For this review, take the finished solid that the model builds, in its own axes (mm). Face numbers are marked on the shaded views. A direction names the side the tool comes from. Give positions to 0.01 mm unless a question says otherwise; leave off trailing zeros. Order: outer loops, then holes, each group sorted by start corner. A loop starts at its lowest first (then second) coordinate and runs counter-clockwise, first axis right, second up. Notation, with made-up numbers: (42.5, -3.5) -> (92.5, -3.5) arc R20 ccw to (92.5, 6.5) -> close; hole circle Ø8 at (74.5, 39). An arc over 180 degrees is marked (long way). Return JSON: item names as keys, results as strings. Group by question number.
1) For the marked faces 1, 2 and 3, list the 3-axis set-ups (+Z, -Z, +X, -X, +Y, -Y) from which the entire face can be reached by the end or side of a thin tool; tool diameter is ignored.
2) Add section A-A (y = 0). State how many separate pieces and enclosed holes the cut face has, then the cut area to 3 significant figures.
3) Add section B-B (x = 0). Give the boundary of the cut face in (y, z) (3 decimals).
4) To check wall thickness, follow line 1 along Y through (x, z) = (0, -9) (3 decimals); line 2 along Y through (x, z) = (10, 16); line 3 along X through (y, z) = (-8, -22). State the ranges of each line that lie inside material, in increasing order.
5) The part is to be moulded in two halves that separate along X. For the marked faces 4, 5, 6 and 7, say which applies: released by +X, released by -X, zero draft, split by the parting line, or undercut.
6) Insertion check: P1, Ø4, axis at x = -29.5, y = 18, coming from the +Z side; P2, Ø14.5, axis at x = 17.46, y = 30.25, coming from the -Z side; P3, Ø1, axis at y = 10, z = 14.5, coming from the -X side. Each pin has a flat end and moves straight along its axis. Give the tip position at first contact, or say it passes through.
from build123d import *

# Parameters (mm, degrees)
F_3_8_0_5_DIAMETER_HOLE1_D = 12.7
CIRPATTERN1_COUNT          = 6


with BuildPart() as part:
    # Sketch1 → Revolve1 (revolve)
    with BuildSketch(Plane(origin=(0, 0, 0), x_dir=(0, 0, -1), z_dir=(1, 0, 0)), mode=Mode.PRIVATE) as revolve1_sk:
        Polygon((-29.3497, 12.7), (29.3497, 12.7), (29.3497, 17.907), (4.826, 22.225), (4.826, 47.625), (22.225, 47.625), (22.225, 50.8), (-22.225, 50.8), (-22.225, 47.625), (-4.826, 47.625), (-4.826, 22.225), (-29.3497, 17.907), align=None)
    revolve(revolve1_sk.sketch.rotate(Axis((0, 0, 50.332885059), (0, 0, -1)), 90), axis=Axis((0, 0, 50.332885059), (0, 0, -1)))

    # 3/8 (0.5) Diameter Hole1 (through all)
    with Locations(Plane.XY.offset(4.826)):
        with Locations((34.925, 0)):
            f_3_8_0_5_diameter_hole1 = Hole(F_3_8_0_5_DIAMETER_HOLE1_D / 2)

    # CirPattern1: 3/8 (0.5) Diameter Hole1 ×6 about axis
    cirpattern1_axis = Axis((0, 0, 0), (0, 0, 1))
    for i in range(1, CIRPATTERN1_COUNT):
        add(f_3_8_0_5_diameter_hole1.rotate(cirpattern1_axis, i * 360 / CIRPATTERN1_COUNT), mode=Mode.SUBTRACT)


solid = part.part
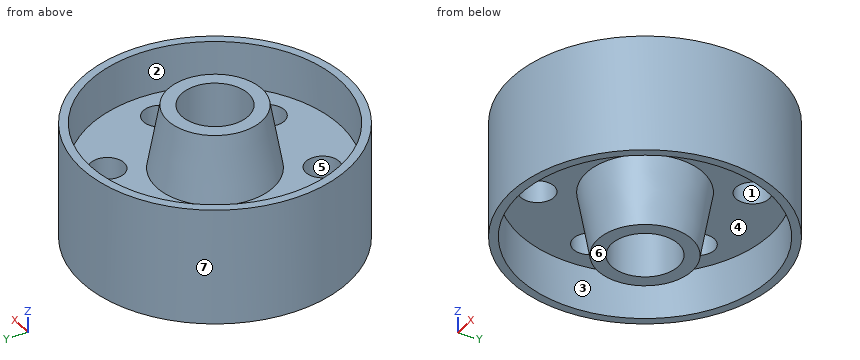
Evaluation:
{
 "1": {"face 1": "+Z, -Z", "face 2": "+Z", "face 3": "-Z"},
 "2": {"separate pieces": "4", "enclosed holes": "0", "area": "1,430 mm^2"},
 "3": {"outline": "(-50.8, -22.225) -> (-47.625, -22.225) -> (-47.625, -4.826) -> (-22.225, -4.826) -> (-17.907, -29.35) -> (-12.7, -29.35) -> (-12.7, 29.35) -> (-17.907, 29.35) -> (-22.225, 4.826) -> (-47.625, 4.826) -> (-47.625, 22.225) -> (-50.8, 22.225) -> close; (12.7, -29.35) -> (17.907, -29.35) -> (22.225, -4.826) -> (47.625, -4.826) -> (47.625, -22.225) -> (50.8, -22.225) -> (50.8, 22.225) -> (47.625, 22.225) -> (47.625, 4.826) -> (22.225, 4.826) -> (17.907, 29.35) -> (12.7, 29.35) -> close"},
 "4": {"line 1": "-50.8 to -47.625, -21.49 to -12.7, 12.7 to 21.49, 47.625 to 50.8", "line 2": "-49.81 to -46.56, -17.62 to -7.83, 7.83 to 17.62, 46.56 to 49.81", "line 3": "-50.17 to -46.95, -17.46 to -9.86, 9.86 to 17.46, 46.95 to 50.17"},
 "5": {"face 4": "undercut", "face 5": "undercut", "face 6": "zero draft", "face 7": "split by the parting line"},
 "6": {"P1": "z = 4.83", "P2": "z = -4.83", "P3": "x = -49.9"}
}
